Work out the finished part from the listing and answer in its coordinate system (mm). Face numbers are marked on the shaded views. A direction names the side the tool comes from. Coordinates: 2 decimals unless noted, no trailing zeros. Order: outer loops, then holes, each group sorted by start corner. A loop starts at its lowest first (then second) coordinate and runs counter-clockwise, first axis right, second up. Notation, with made-up numbers: (63.5, -7.5) -> (93.5, -7.5) arc R11 ccw to (93.5, 8.5) -> close; hole circle Ø6 at (21.25, 81). An arc over 180 degrees is marked (long way). Use one line per item in the form item = value.
from build123d import *

# Parameters (mm, degrees)
SKETCH_1_R      = 4
EXTRUDE_1_DEPTH = 60
SKETCH_2_W      = 40
SKETCH_2_H      = 3
REVOLVE_1_ANGLE = 90
SKETCH_3_W      = 40
SKETCH_3_H      = 3
REVOLVE_2_ANGLE = 90


with BuildPart() as part:
    # 草图1 → 凸台-拉伸1 (new body)
    with BuildSketch(Plane.XY):
        Circle(SKETCH_1_R)
    extrude(amount=EXTRUDE_1_DEPTH)

    # 草图2 → 旋转1 (revolve)
    with BuildSketch(Plane(origin=(0, 0, 0), x_dir=(1, 0, 0), z_dir=(0, 1, 0))):
        with Locations((20, -49.5)):
            Rectangle(SKETCH_2_W, SKETCH_2_H)
    revolve(axis=Axis((0, 0, -2.761338376), (0, 0, 1)), revolution_arc=REVOLVE_1_ANGLE)

    # 草图3 → 旋转2 (revolve)
    with BuildSketch(Plane(origin=(0, 0, 0), x_dir=(1, 0, 0), z_dir=(0, 1, 0))):
        with Locations((20, -1.5)):
            Rectangle(SKETCH_3_W, SKETCH_3_H)
    revolve(axis=Axis((0, 0, -6.370265632), (0, 0, -1)), revolution_arc=REVOLVE_2_ANGLE)


solid = part.part
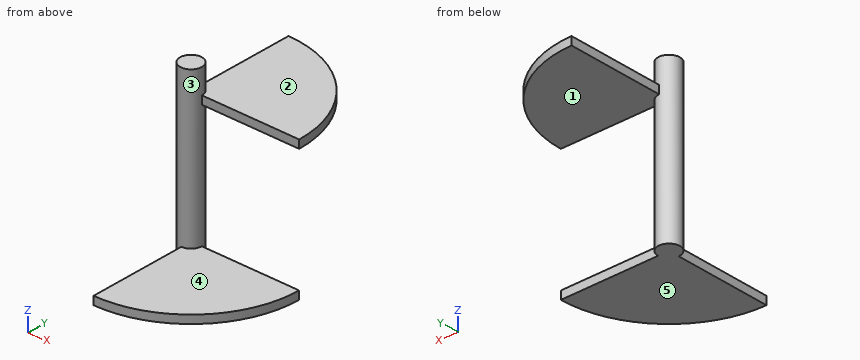
(1) Each of these flat-tipped pins is pushed along its axis until it touches: P1, Ø12, axis at x = 32, y = 20, coming from the -Z side; P2, Ø3.5, axis at y = -16.5, z = 1.5, coming from the -X side; P3, Ø6, axis at x = 0.5, z = 40.5, coming from the +Y side. Where does it stop, or does it pass through?
Data:
P1 = 48
P2 = 0
P3 = 4
(2) Section A-A on x = 27.5 is taken. Write down the section's boundary in (y, z), plus the area to 3 significant figures.
Data:
outline = (-29.05, 0) -> (0, 0) -> (0, 3) -> (-29.05, 3) -> close; (0, 48) -> (29.05, 48) -> (29.05, 51) -> (0, 51) -> close
area = 174 mm²
(3) Section B-B on z = 31 is taken. Write down the section's boundary in (x, y).
Data:
outline = circle Ø8 at (0, 0)
(4) Straight lines are drawn through the part: line 1 along Z through (x, y) = (12, 7); line 2 along Z through (x, y) = (6, -14); line 3 along X through (y, z) = (-2, 8). For each, find the intervals that lie inside material, in ascending order.
Data:
line_1 = 48 to 51
line_2 = 0 to 3
line_3 = -3.46 to 3.46
(5) Which of the six approach directions +Z, -Z, +X, -X, +Y, -Y give full straight-line access (tool end or side, diameter ignored) to the marked faces 1, 2, 3, 4 and 5?
Data:
face_1 = -Z, +X, +Y
face_2 = +Z, +X, +Y
face_3 = none
face_4 = +Z, +X, -Y
face_5 = -Z, +X, -X, +Y, -Y
(6) Section C-C on y = -24 is taken. Write down the section's boundary in (x, z).
Data:
outline = (0, 0) -> (32, 0) -> (32, 3) -> (0, 3) -> close
(7) Section D-D on x = 11.5 is taken. Write down the section's boundary in (y, z).
Data:
outline = (-38.31, 0) -> (0, 0) -> (0, 3) -> (-38.31, 3) -> close; (0, 48) -> (38.31, 48) -> (38.31, 51) -> (0, 51) -> close
